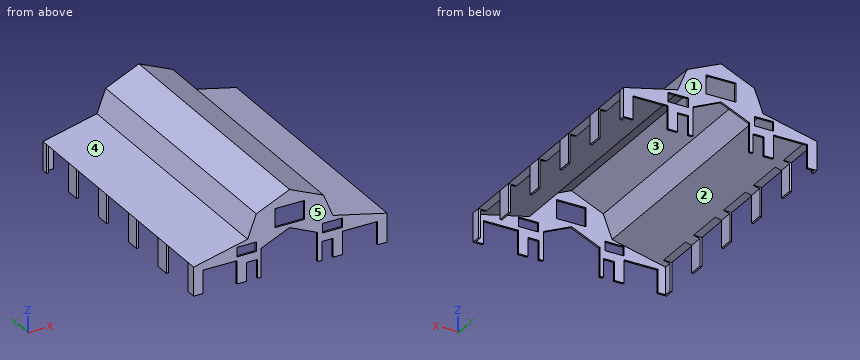
from build123d import *

# Parameters (mm, degrees)
F1_DEPTH = 351.282
F2_T     = -2.54
F3_W     = 40.0430839509
F3_H     = 25.3932625055
F3_W_2   = 14.9065516889
F3_H_2   = 25.1731947064
F4_DEPTH = 508
F5_W     = 50.8
F5_H     = 38.6911868118
F6_DEPTH = 558.8
F7_W     = 45.9006593287
F7_H     = 31.1064030975
F7_W_2   = 25.9576785982
F7_H_2   = 12.7
F7_W_3   = 27.178
F7_W_4   = 47.3086998522
F8_DEPTH = 762


with BuildPart() as f1:
    # F0 (on Front) → F1 (new body)
    with BuildSketch(Plane.XZ):
        Polygon((-44.8798835278, 55.2486851811), (-56.6415078938, 24.6065575629), (-129.4382214546, 7.5847837143), (-129.4382214546, -31.1064030975), (131.4852535725, -31.1064030975), (131.4852535725, 7.5847837143), (58.4986023605, 24.6065575629), (45.8084307611, 55.2486851811), (0, 75.367256999), align=None)
    extrude(amount=-F1_DEPTH)

    # F2
    f2_openings = [f1.faces().sort_by_distance(p)[0] for p in [
        (1.023516, 175.641, -31.106403),
    ]]
    offset(amount=F2_T, openings=f2_openings, kind=Kind.INTERSECTION)

    # F3 (on face) → F4 (cut)
    with BuildSketch(Plane(origin=(0, 351.282, 0), x_dir=(-1, 0, 0), z_dir=(0, 1, 0))):
        with Locations((-0.1733517274, 42.5520539284)):
            Rectangle(F3_W, F3_H)
        with Locations((50.6842862815, -18.5198057443)):
            Rectangle(F3_W_2, F3_H_2)
        with Locations((-51.3232778758, -18.5198057443)):
            Rectangle(F3_W_2, F3_H_2)
        Polygon((-38.0242951214, -31.1064030975), (0, -31.1064030975), (38.2621623576, -31.1064030975), (38.2621623576, 7.5847837143), (0, 24.6065575629), (-38.0242951214, 7.5847837143), align=None)
    extrude(amount=-F4_DEPTH, mode=Mode.SUBTRACT)

    # F5 (on face) → F6 (cut)
    with BuildSketch(Plane.YZ.offset(131.4852535725)):
        with Locations((38.1, -11.7608096916)):
            Rectangle(F5_W, F5_H)
        with Locations((107.95, -11.7608096916)):
            Rectangle(F5_W, F5_H)
        with Locations((177.8, -11.7608096916)):
            Rectangle(F5_W, F5_H)
        with Locations((247.65, -11.7608096916)):
            Rectangle(F5_W, F5_H)
        with Locations((317.5, -11.7608096916)):
            Rectangle(F5_W, F5_H)
    extrude(amount=-F6_DEPTH, mode=Mode.SUBTRACT)

    # F7 (on face) → F8 (cut)
    with BuildSketch(Plane.XZ):
        with Locations((-93.7878917903, -15.5532015488)):
            Rectangle(F7_W, F7_H)
        with Locations((-57.8587228268, 11.43)):
            Rectangle(F7_W_2, F7_H_2)
        with Locations((57.8875537202, 11.43)):
            Rectangle(F7_W_3, F7_H_2)
        with Locations((95.1309036463, -15.5532015488)):
            Rectangle(F7_W_4, F7_H)
    extrude(amount=-F8_DEPTH, mode=Mode.SUBTRACT)


solid = f1.part
Geometry check sheet. Reference: the model listing, model coordinates, mm. Face numbers are marked on the shaded views. A direction names the side the tool comes from. Give positions to 0.01 mm unless a question says otherwise; leave off trailing zeros. Loops run counter-clockwise (first coordinate to the right, second up) from the corner with the lowest first, then second, coordinate; pieces in that order, holes last. Notation, with made-up numbers: (66, -39) -> (97, -39) arc R18 ccw to (97, -19) -> close; hole circle Ø1 at (81, -7.75). An arc over 180 degrees is marked (long way). Answer in a Markdown table with one row per item. Add a question column.
1) Draft check along Y on the marked faces 3, 4 and 5. Enter one of: pulls with the +Y half, pulls with the -Y half, needs draft (parallel to the pull), parting line crosses it, or undercut.
2) Cross-section at A-A on y = 218. Record the boundary of the cut face in (x, z).
3) Cross-section at C-C on z = 64.5. Record the boundary of the cut face in (x, y).
4) Set-up check for the marked faces 1 and 2: record each of +Z, -Z, +X, -X, +Y, -Y from which the full face is reachable in a straight line by a thin tool's end or side.
5) Cross-section at D-D on x = 81. Record the boundary of the cut face in (y, z), and give its area (3 significant figures).
6) Cross-section at B-B on x = 52.5. Record the boundary of the cut face in (y, z), and give its area (3 significant figures).
7) Gauge pin test, flat ends, axial feed: P1, Ø12, axis at x = -34.5, y = 290, coming from the +Z side; P2, Ø1.5, axis at x = -3.5, y = 97.5, coming from the +Z side; P3, Ø0.8, axis at x = 51.5, y = 350, coming from the -Z side. Record the tip position at first contact, or that the pin passes through.
8) Material ranges on probe 1 along Y at (x, z) = (-3.5, 58.5); probe 2 along X at (y, z) = (147.5, 55); probe 3 along X at (y, z) = (277, 45), recorded low to high. Write a range as from..to.
Outcome:
| question | item | result |
|---|---|---|
| 1 | face 3 | undercut |
| 1 | face 4 | needs draft |
| 1 | face 5 | pulls with the -Y half |
| 2 | outline | (-129.44, -31.11) -> (-126.9, -31.11) -> (-126.9, 5.57) -> (-54.75, 22.44) -> (-42.88, 53.36) -> (0.01, 72.59) -> (43.85, 53.33) -> (56.65, 22.43) -> (128.95, 5.57) -> (128.95, -31.11) -> (131.49, -31.11) -> (131.49, 7.58) -> (58.5, 24.61) -> (45.81, 55.25) -> (0, 75.37) -> (-44.88, 55.25) -> (-56.64, 24.61) -> (-129.44, 7.58) -> close |
| 3 | outline | (-24.24, 0) -> (24.74, 0) -> (24.74, 351.28) -> (-24.24, 351.28) -> close; hole (-18.03, 2.54) -> (18.43, 2.54) -> (18.43, 348.74) -> (-18.03, 348.74) -> close |
| 4 | face 1 | +Z, -Z, +X, -X, +Y |
| 4 | face 2 | -Z |
| 5 | outline | (0, 0) -> (2.54, 0) -> (2.54, 16.75) -> (348.74, 16.75) -> (348.74, 0) -> (351.28, 0) -> (351.28, 19.36) -> (0, 19.36) -> close |
| 5 | area | 1,000 mm^2 |
| 6 | outline | (0, -5.93) -> (2.54, -5.93) -> (2.54, 5.08) -> (0, 5.08) -> close; (0, 17.78) -> (2.54, 17.78) -> (2.54, 32.45) -> (348.74, 32.45) -> (348.74, 17.78) -> (351.28, 17.78) -> (351.28, 39.09) -> (0, 39.09) -> close; (348.74, -5.93) -> (351.28, -5.93) -> (351.28, 5.08) -> (348.74, 5.08) -> close |
| 6 | area | 2,460 mm^2 |
| 7 | P1 | stops at z = 62.59 |
| 7 | P2 | stops at z = 74.13 |
| 7 | P3 | stops at z = -5.93 |
| 8 | probe 1 | y = 0..2.54, 348.74..351.28 |
| 8 | probe 2 | x = -44.98..-39.23, 40.06..45.91 |
| 8 | probe 3 | x = -48.81..-46.09, 47.3..50.05 |
